Geometry check sheet. Reference: the model listing, model coordinates, mm. Face numbers are marked on the shaded views. Give positions to 0.01 mm unless a question says otherwise; leave off trailing zeros. Loops run counter-clockwise (first coordinate to the right, second up) from the corner with the lowest first, then second, coordinate; pieces in that order, holes last.
1. Cross-section at B-B, the plane z = 3. Record the cut outline in (x, y).
2. Go/stop test with a flat-tipped pin: pin 1 Ø4.5 at (x, y) = (4, 68) entering from -Z. Record where the tip stops, or that it passes through.
3. Release check for a two-part mould opening along X. For the marked faces 1, 2, 3 and 4 record: +X half, -X half, draft (parallel to the pull), parting line (faces both ways), or undercut.
4. Material ranges on L1, parallel to Y at x = 4.25, z = 5.5; L2, parallel to Y at x = 4.5, z = 3.5; L3, parallel to Z at x = 7.5, y = 65, recorded low to high.
5. Cross-section at C-C, the plane x = 4. State how many separate pieces and enclosed holes the cut face has, plus the area to 3 significant figures.
Autodesk Inventor part; units mm, degrees
ref_plane "YZ Plane" through (0, 0, 0) normal (1, 0, 0) x (0, 1, 0)
ref_plane "XZ Plane" through (0, 0, 0) normal (0, 1, 0) x (-1, 0, 0)
ref_plane "XY Plane" through (0, 0, 0) normal (0, 0, 1) x (1, 0, 0)
sketch "Sketch1" plane through (0, 0, 0) normal (0, 0, 1) x (1, 0, 0)
  line L0 (0, 72) -> (8, 72)
  line L1 (8, 72) -> (8, 0)
  line L2 (8, 0) -> (0, 0)
  line L3 (0, 0) -> (0, 72)
  circle A0 centre (4, 68) radius 2.5
  circle A1 centre (4, 4) radius 2.5
  dimension "d0" = 8
  dimension "d1" = 72
  dimension "d2" = 5
  dimension "d3" = 5
  dimension "d4" = 4
  dimension "d5" = 64
  dimension "d7" = 4
  dimension "d8" = 4
extrude "Extrusion1" add sketch "Sketch1" along normal blind 8
fillet "Fillet1" radius 3 4 edges at (8, 72, 4) (0, 72, 4) (8, 0, 4) (0, 0, 4)
chamfer "Chamfer1" distance 1.5 angle 45 16 edges at (0, 36, 8) (0.8787, 0.8787, 8) (4, 0, 8) (7.1213, 0.8787, 8) (8, 36, 8) (7.1213, 71.1213, 8) (4, 72, 8) (0.8787, 71.1213, 8) (8, 36, 0) (7.1213, 71.1213, 0) (4, 72, 0) (0.8787, 71.1213, 0) (0, 36, 0) (0.8787, 0.8787, 0) (4, 0, 0) (7.1213, 0.8787, 0)
equation "\"d3\" = d2"
properties part number "base"
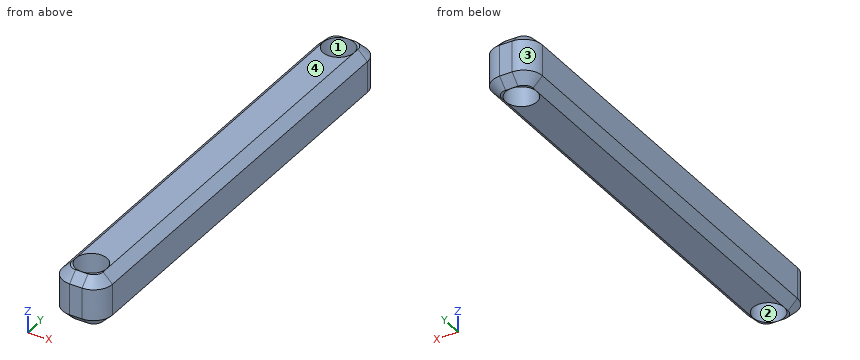
Result:
1. outline: (0, 3) arc R3 ccw to (3, 0) - (5, 0) arc R3 ccw to (8, 3) - (8, 69) arc R3 ccw to (5, 72) - (3, 72) arc R3 ccw to (0, 69) - close; hole circle Ø5 at (4, 4); hole circle Ø5 at (4, 68)
2. pin 1: passes through
3. face 1: undercut
3. face 2: undercut
3. face 3: -X half
3. face 4: draft
4. L1: y = 0 to 1.51, 6.49 to 65.51, 70.49 to 72
4. L2: y = 0 to 1.55, 6.45 to 65.55, 70.45 to 72
4. L3: z = 1 to 7
5. separate pieces: 3
5. enclosed holes: 0
5. area: 492 mm2
